Geometry check sheet. Reference: the model listing, model coordinates, mm. Round coordinates to 2 decimals unless told otherwise and drop trailing zeros. Loops run counter-clockwise (first coordinate to the right, second up) from the corner with the lowest first, then second, coordinate; pieces in that order, holes last. Notation, with made-up numbers: (56, 36.25) - (67, 36.25) arc R24 ccw to (67, 66.25) - close; hole circle Ø2 at (-3, 69). An arc over 180 degrees is marked (long way). Answer as CSV lines item,"result". Start each with the question number.
1) Cross-section at B-B on y = 76.5. Record the boundary of the cut face in (x, z), and give its area (3 significant figures).
2) Cross-section at C-C on x = -157. Record the boundary of the cut face in (y, z).
3) Depth check by flat-ended pin: P1, Ø1.8, axis at x = -253.42, y = 140.98, coming from the -Z side; P2, Ø1.5, axis at y = 192, z = 3.5, coming from the +X side; P3, Ø1, axis at y = 142.5, z = 3, coming from the +X side. Enter the tip coordinate at first touch or a pass-through.
4) Thickness scan on line 1 along Y through (x, z) = (-267, 3.1); line 2 along Y through (x, z) = (-208, 2.1); line 3 along X through (y, z) = (49, 1.35). Record the ranges inside material, lowest first.
5) Draft check along Y on faces 1 (the cylindrical face through (-226.11, 128.35, 1.97)), 2 (the flat face through (-234, 140, 0)), 3 (the cylindrical face through (-260.9, 148.09, 1.97)). Enter one of: released by +Y, released by -Y, zero draft, split by the parting line, or undercut.
6) Cross-section at A-A on z = 1.7. State how many separate pieces and enclosed holes the cut face has, and give its area (3 significant figures).
Autodesk Inventor part; units mm, degrees
ref_plane "YZ Plane" through (0, 0, 0) normal (1, 0, 0) x (0, 1, 0)
ref_plane "XZ Plane" through (0, 0, 0) normal (0, 1, 0) x (-1, 0, 0)
ref_plane "XY Plane" through (0, 0, 0) normal (0, 0, 1) x (1, 0, 0)
sketch "Sketch1" plane through (0, 0, 0) normal (0, 0, 1) x (1, 0, 0)
  circle A0 centre (0, 0) radius 260
  circle A1 centre (0, 0) radius 300
  dimension "d0" = 600
  dimension "d1" = 40
extrude "Extrusion1" add sketch "Sketch1" along normal blind 4
sketch "Sketch2" plane through (0, 0, 4) normal (0, 0, 1) x (1, 0, 0)
  line L0 (300, 35.8531) -> (300, -300)
  line L1 (300, -300) -> (-300, -300)
  line L2 (-300, -300) -> (-300, 0)
  circle A0 centre (0, 0) radius 300
  line L3 (-420, 0) -> (420, 0)
  circle A1 centre (0, 0) radius 300
  line L4 (-300, 0) -> (0, 0)
  line L5 (0, 0) -> (-150, 259.8076)
  line L6 (-150, 259.8076) -> (-150, 300)
  line L7 (-150, 300) -> (300, 300)
  line L8 (300, 300) -> (300, 35.8531)
  dimension "d25" = 60
extrude "Extrusion2" cut sketch "Sketch2" against normal blind 10 contours L3 L5 A0 | A0 L3 picked at (97.6489, 174.3647)
sketch "Sketch3" plane through (0, 0, 4) normal (0, 0, 1) x (1, 0, 0)
  circle A0 centre (-287.9915, 36.5258) radius 1.5
  circle A1 centre (-266.6759, 42.2373) radius 1.5
  line L0 (-420, 0) -> (420, 0)
  circle A2 centre (-286.355, 45.8069) radius 1.5
  circle A3 centre (-265.0393, 51.5184) radius 1.5
  line L1 (-266.6759, 42.2373) -> (-287.9915, 36.5258)
  line L2 (-287.9915, 36.5258) -> (-286.355, 45.8069)
  line L3 (-286.355, 45.8069) -> (-265.0393, 51.5184)
  line L4 (-265.0393, 51.5184) -> (-266.6759, 42.2373)
  line L5 (-265.0393, 51.5184) -> (0, 0)
  line L6 (0, 0) -> (-266.6759, 42.2373)
  dimension "d6" = 3
  dimension "d7" = 3
  dimension "d9" = 270
  dimension "d11" = 3
  dimension "d12" = 3
  dimension "d14" = 270
  dimension "d21" = 115
  dimension "d22" = 20
  dimension "d23" = 9
  dimension "d24" = 11
extrude "Extrusion3" cut sketch "Sketch3" against normal through all contours A0 L2 L1 | L1 L2 A0 | L1 L6 A1 | A1 L4 L1 | L2 L3 A2 | A2 L3 L2 | A1 L6 L4 | L4 L5 A3 | A3 L3 L4 | A3 L5 L3
pattern_circular "Circular Pattern1" count 9 over 160 about axis through (0, 0, 0) along (0, 0, -1) of "Extrusion3"
properties part number "wheel7"
Answer block:
1,outline,"(-290.08, 0) - (-248.49, 0) - (-248.49, 4) - (-290.08, 4) - close"
1,area,"166 mm^2"
2,outline,"(207.25, 0) - (255.64, 0) - (255.64, 4) - (207.25, 4) - close"
3,P1,"passes through"
3,P2,"stops at x = -174.49"
3,P3,"stops at x = -217.14"
4,line 1,"y = 0 to 40.77, 43.7 to 136.79"
4,line 2,"y = 156 to 216.19"
4,line 3,"x = -295.97 to -255.34"
5,face 1,"released by -Y"
5,face 2,"zero draft"
5,face 3,"released by +Y"
6,separate pieces,"1"
6,enclosed holes,"12"
6,area,"11,700 mm^2"
